For this review, take the finished solid that the model builds, in its own axes (mm). Face numbers are marked on the shaded views. A direction names the side the tool comes from. Give positions to 0.01 mm unless a question says otherwise; leave off trailing zeros. Order: outer loops, then holes, each group sorted by start corner. A loop starts at its lowest first (then second) coordinate and runs counter-clockwise, first axis right, second up. Notation, with made-up numbers: (-9, 42) -> (42, 42) arc R11 ccw to (42, 48) -> close; hole circle Ø8 at (36.5, 54). An arc over 180 degrees is marked (long way). Use CSV: the item, a comma, the result in double quotes. Start each with the question number.
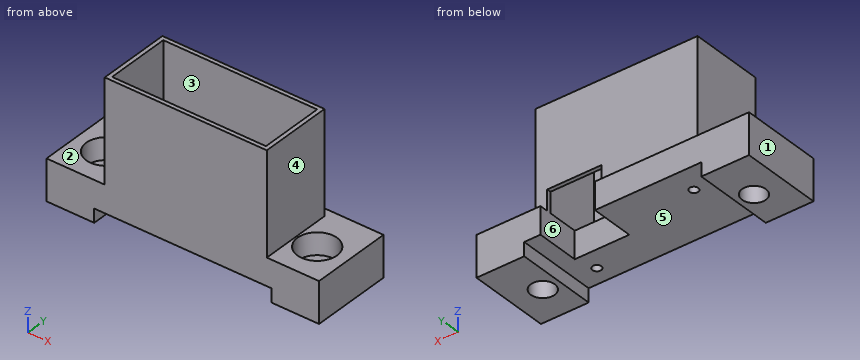
```python
from build123d import *

# Parameters (mm, degrees)
SKETCH4_W               = 50.8
SKETCH4_H               = 16.764
BOSS_EXTRUDE1_DEPTH     = 7.62
SKETCH5_R               = 0.8255
SKETCH5_W               = 10.16
SKETCH5_H               = 5.08
CUT_EXTRUDE1_DEPTH      = 7.62
SKETCH6_R               = 3.683
SKETCH6_R_2             = 2.2225
CUT_EXTRUDE2_DEPTH      = 4.064
SKETCH6_2_R             = 2.2225
CUT_EXTRUDE3_DEPTH      = 7.62
SKETCH7_W               = 33.02
SKETCH7_H               = 5.08
CUT_EXTRUDE4_DEPTH      = 1
CUT_EXTRUDE4_DEPTH_BACK = 17.764
SKETCH8_W               = 10.16
SKETCH8_H               = 2.54
CUT_EXTRUDE5_DEPTH      = 4.064
SKETCH9_W               = 30.2133
SKETCH9_H               = 13.5763
SKETCH9_W_2             = 28.6893
SKETCH9_H_2             = 12.0523
BOSS_EXTRUDE4_DEPTH     = 19.05
SKETCH12_W              = 10.16
SKETCH12_H              = 2.99085
CUT_EXTRUDE6_DEPTH      = 6.35
SKETCH13_W              = 50.8
SKETCH13_H              = 1.59385
CUT_EXTRUDE7_DEPTH      = 20.05
CUT_EXTRUDE7_DEPTH_BACK = 8.62


with BuildPart() as part:
    # Sketch4 → Boss-Extrude1 (new body)
    with BuildSketch(Plane.XY):
        Rectangle(SKETCH4_W, SKETCH4_H)
    extrude(amount=BOSS_EXTRUDE1_DEPTH)

    # Sketch5 → Cut-Extrude1 (cut)
    with BuildSketch(Plane.XY.offset(7.62)):
        with Locations((-11.24585, 3.48615)):
            Circle(SKETCH5_R)
        with Locations((12.36345, -3.48615)):
            Circle(SKETCH5_R)
        with Locations((8.40105, 2.85115)):
            Rectangle(SKETCH5_W, SKETCH5_H)
    extrude(amount=-CUT_EXTRUDE1_DEPTH, mode=Mode.SUBTRACT)

    # Sketch6 → Cut-Extrude2 (cut)
    with BuildSketch(Plane.XY.offset(7.62)):
        with Locations((-19.685, 0)):
            Circle(SKETCH6_R)
        with Locations((-19.685, 0)):
            Circle(SKETCH6_R_2, mode=Mode.SUBTRACT)
        with Locations((19.685, 0)):
            Circle(SKETCH6_R)
        with Locations((19.685, 0)):
            Circle(SKETCH6_R_2, mode=Mode.SUBTRACT)
    extrude(amount=-CUT_EXTRUDE2_DEPTH, mode=Mode.SUBTRACT)

    # Sketch6_2 → Cut-Extrude3 (cut)
    with BuildSketch(Plane.XY.offset(7.62)):
        with Locations((-19.685, 0)):
            Circle(SKETCH6_2_R)
        with Locations((19.685, 0)):
            Circle(SKETCH6_2_R)
    extrude(amount=-CUT_EXTRUDE3_DEPTH, mode=Mode.SUBTRACT)

    # Sketch7 → Cut-Extrude4 (cut, two sides)
    with BuildSketch(Plane(origin=(0, 8.382, 0), x_dir=(1, 0, 0), z_dir=(0, 1, 0))) as cut_extrude4_sk:
        Rectangle(SKETCH7_W, SKETCH7_H)
    extrude(amount=CUT_EXTRUDE4_DEPTH, mode=Mode.SUBTRACT)
    extrude(cut_extrude4_sk.sketch, amount=-CUT_EXTRUDE4_DEPTH_BACK, mode=Mode.SUBTRACT)

    # Sketch8 → Cut-Extrude5 (cut)
    with BuildSketch(Plane.XZ.offset(-5.39115)):
        with Locations((8.40105, 3.81)):
            Rectangle(SKETCH8_W, SKETCH8_H)
    extrude(amount=-CUT_EXTRUDE5_DEPTH, mode=Mode.SUBTRACT)

    # Sketch9 → Boss-Extrude4 (add)
    with BuildSketch(Plane.XY.offset(7.62)):
        with Locations((0.5588, 0)):
            Rectangle(SKETCH9_W, SKETCH9_H)
        with Locations((0.5588, 0)):
            Rectangle(SKETCH9_W_2, SKETCH9_H_2, mode=Mode.SUBTRACT)
    extrude(amount=BOSS_EXTRUDE4_DEPTH)

    # Sketch12 → Cut-Extrude6 (cut)
    with BuildSketch(Plane(origin=(0, 0, 5.08), x_dir=(-1, 0, 0), z_dir=(0, 0, -1))):
        with Locations((-8.40105, 6.886575)):
            Rectangle(SKETCH12_W, SKETCH12_H)
    extrude(amount=-CUT_EXTRUDE6_DEPTH, mode=Mode.SUBTRACT)

    # Sketch13 → Cut-Extrude7 (cut, two sides)
    with BuildSketch(Plane.XY.offset(7.62)) as cut_extrude7_sk:
        with Locations((0, -7.585075)):
            Rectangle(SKETCH13_W, SKETCH13_H)
    extrude(amount=CUT_EXTRUDE7_DEPTH, mode=Mode.SUBTRACT)
    extrude(cut_extrude7_sk.sketch, amount=-CUT_EXTRUDE7_DEPTH_BACK, mode=Mode.SUBTRACT)


solid = part.part
```
1. Clearance check with flat-ended pins moving along their axes: P1, Ø6, axis at x = 19.685, y = 0, coming from the +Z side; P2, Ø1, axis at x = -19.5, y = -1.5, coming from the +Z side; P3, Ø4, axis at x = 10, z = 5, coming from the +Y side; P4, Ø7, axis at y = 1, z = 14, coming from the +X side. State where each tip first meets the part, or that it passes through.
2. Consider section B-B (z = 13.5). State the section outline as (x, y) points.
3. Draft analysis for pull direction X (two halves, no side actions). For the marked faces 1, 2 and 3, state which applies: +X half, -X half, draft (parallel to the pull), parting line (faces both ways), or undercut.
4. Consider section C-C (x = -9). State the section outline as (y, z) points.
5. Consider section D-D (y = -1). State how many separate pieces and enclosed holes the cut face has, plus the area to 3 significant figures.
6. Consider section A-A (y = 5.5). State the section outline as (x, z) points, plus the area to 3 significant figures.
7. For the marked faces 4, 5 and 6, list the 3-axis set-ups (+Z, -Z, +X, -X, +Y, -Y) from which the entire face can be reached by the end or side of a thin tool; tool diameter is ignored.
8. To check wall thickness, follow L1, parallel to Y at x = -12, z = 19.25; L2, parallel to X at y = 5.5, z = 19.5; L3, parallel to X at y = 6.75, z = 8. State the ranges of each line that lie inside material, in increasing order. Write a range as [from, to].
Answer list:
1,P1,"z = 3.56"
1,P2,"through"
1,P3,"y = 0.31"
1,P4,"x = 15.67"
2,outline,"(-14.55, -6.79) -> (15.67, -6.79) -> (15.67, 6.79) -> (-14.55, 6.79) -> close; hole (-13.79, -6.03) -> (14.9, -6.03) -> (14.9, 6.03) -> (-13.79, 6.03) -> close"
3,face 1,"-X half"
3,face 2,"draft"
3,face 3,"undercut"
4,outline,"(-6.79, 2.54) -> (8.38, 2.54) -> (8.38, 7.62) -> (6.79, 7.62) -> (6.79, 26.67) -> (6.03, 26.67) -> (6.03, 7.62) -> (-6.03, 7.62) -> (-6.03, 26.67) -> (-6.79, 26.67) -> close"
5,separate pieces,"3"
5,enclosed holes,"0"
5,area,"246 mm2"
6,outline,"(-25.4, 0) -> (-16.51, 0) -> (-16.51, 2.54) -> (3.32, 2.54) -> (3.32, 7.62) -> (-13.79, 7.62) -> (-13.79, 26.67) -> (-14.55, 26.67) -> (-14.55, 7.62) -> (-25.4, 7.62) -> close; (13.48, 2.54) -> (16.51, 2.54) -> (16.51, 0) -> (25.4, 0) -> (25.4, 7.62) -> (15.67, 7.62) -> (15.67, 26.67) -> (14.9, 26.67) -> (14.9, 7.62) -> (13.48, 7.62) -> close"
6,area,"281 mm2"
7,face 4,"+Z, +X, +Y, -Y"
7,face 5,"-Z, +Y, -Y"
7,face 6,"-Z, +Y"
8,L1,"[-6.79, -6.03], [6.03, 6.79]"
8,L2,"[-14.55, -13.79], [14.9, 15.67]"
8,L3,"[-14.55, 3.32], [13.48, 15.67]"
